Autodesk Inventor part; units mm, degrees
ref_plane "YZ Plane" through (0, 0, 0) normal (1, 0, 0) x (0, 1, 0)
ref_plane "XZ Plane" through (0, 0, 0) normal (0, 1, 0) x (-1, 0, 0)
ref_plane "XY Plane" through (0, 0, 0) normal (0, 0, 1) x (1, 0, 0)
sketch "Sketch3" plane through (0, 0, 0) normal (0, 1, 0) x (-1, 0, 0)
  circle A0 centre (0, 0) radius 13.5
  line L0 (-6.7499, 8.6501) -> (-1.7499, 8.6501)
  line L1 (-1.7499, 8.6501) -> (-1.7499, 7.1501)
  line L2 (-1.7499, 7.1501) -> (-6.7499, 7.1501)
  line L3 (-6.7499, 7.1501) -> (-6.7499, 8.6501)
  line L4 (-6.75, 5.45) -> (-1.7499, 5.45)
  line L5 (-1.7499, 5.45) -> (-1.7499, 3.95)
  line L6 (-1.7499, 3.95) -> (-6.75, 3.95)
  line L7 (-6.75, 3.95) -> (-6.75, 5.45)
  line L8 (-6.75, 2.0498) -> (-1.75, 2.0498)
  line L9 (-1.75, 2.0498) -> (-1.75, 0.5498)
  line L10 (-1.75, 0.5498) -> (-6.75, 0.5498)
  line L11 (-6.75, 0.5498) -> (-6.75, 2.0498)
  line L12 (-6.75, -1.2) -> (-1.75, -1.2)
  line L13 (-1.75, -1.2) -> (-1.75, -2.7)
  line L14 (-1.75, -2.7) -> (-6.75, -2.7)
  line L15 (-6.75, -2.7) -> (-6.75, -1.2)
  line L16 (-6.75, -4.4501) -> (-1.75, -4.4501)
  line L17 (-1.75, -4.4501) -> (-1.75, -5.9501)
  line L18 (-1.75, -5.9501) -> (-6.75, -5.9501)
  line L19 (-6.75, -5.9501) -> (-6.75, -4.4501)
  line L20 (1.9499, 7.1) -> (6.9499, 7.1)
  line L21 (6.9499, 7.1) -> (6.9499, 5.6)
  line L22 (6.9499, 5.6) -> (1.9499, 5.6)
  line L23 (1.9499, 5.6) -> (1.9499, 7.1)
  line L24 (1.9499, 3.95) -> (6.9499, 3.95)
  line L25 (6.9499, 3.95) -> (6.9499, 2.45)
  line L26 (6.9499, 2.45) -> (1.9499, 2.45)
  line L27 (1.9499, 2.45) -> (1.9499, 3.95)
  line L28 (1.9499, 0.5004) -> (6.9499, 0.5004)
  line L29 (6.9499, 0.5004) -> (6.9499, -0.9996)
  line L30 (6.9499, -0.9996) -> (1.9499, -0.9996)
  line L31 (1.9499, -0.9996) -> (1.9499, 0.5004)
  line L32 (1.9499, -2.7) -> (6.9499, -2.7)
  line L33 (6.9499, -2.7) -> (6.9499, -4.2)
  line L34 (6.9499, -4.2) -> (1.9499, -4.2)
  line L35 (1.9499, -4.2) -> (1.9499, -2.7)
  line L36 (1.9499, -6.1999) -> (6.9499, -6.1999)
  line L37 (6.9499, -6.1999) -> (6.9499, -7.6999)
  line L38 (6.9499, -7.6999) -> (1.9499, -7.6999)
  line L39 (1.9499, -7.6999) -> (1.9499, -6.1999)
  point P0 (-6.7499, 7.9001)
  point P1 (-6.75, 4.7)
  point P2 (-5.95, -5.2001)
  dimension "d3" = 27
  dimension "d4" = 5
  dimension "d5" = 1.5
  dimension "d6" = 1.5
  dimension "d7" = 5
  dimension "d8" = 1.5
  dimension "d9" = 5
  dimension "d10" = 1.5
  dimension "d11" = 5
  dimension "d12" = 1.5
  dimension "d13" = 0.8
  dimension "d14" = 5
  dimension "d15" = 1.5
  dimension "d16" = 5
  dimension "d17" = 1.5
  dimension "d18" = 5
  dimension "d19" = 1.5
  dimension "d20" = 5
  dimension "d21" = 1.5
  dimension "d22" = 1.5
extrude "Extrusion1" add sketch "Sketch3" along normal blind 5
sketch "Sketch4" plane through (0, 5, 0) normal (0, 1, 0) x (1, 0, 0)
  circle A0 centre (-10.8, -1.9) radius 0.75
  circle A1 centre (-10.8, 1.7) radius 0.75
  circle A2 centre (10.9, -1.85) radius 0.75
  circle A3 centre (10.9, 1.65) radius 0.75
  circle A4 centre (0.958, 9.985) radius 3
  point P0 (0, 0)
  dimension "d25" = 1.5
  dimension "d26" = 1.5
  dimension "d27" = 1.5
  dimension "d28" = 1.5
  dimension "d29" = 6
extrude "Extrusion2" cut sketch "Sketch4" against normal blind 5
sketch "Sketch5" plane through (0, 5, 0) normal (0, 1, 0) x (1, 0, 0)
  circle A0 centre (-10.8, -1.9) radius 0.75
  circle A1 centre (-10.8, -1.9) radius 1.25
  circle A2 centre (-10.8, 1.7) radius 0.75
  circle A3 centre (-10.8, 1.7) radius 1.25
  circle A4 centre (10.9, -1.85) radius 0.75
  circle A5 centre (10.9, -1.85) radius 1.25
  circle A6 centre (10.9, 1.65) radius 0.75
  circle A7 centre (10.9, 1.65) radius 1.25
  point P0 (0, 0)
  dimension "d33" = 2.5
  dimension "d34" = 2.5
  dimension "d35" = 2.5
  dimension "d36" = 2.5
extrude "Extrusion3" cut sketch "Sketch5" against normal blind 5 contours A0 | A1 | A2 | A3 | A4 | A5 | A6 | A7
properties part number "Seperator"
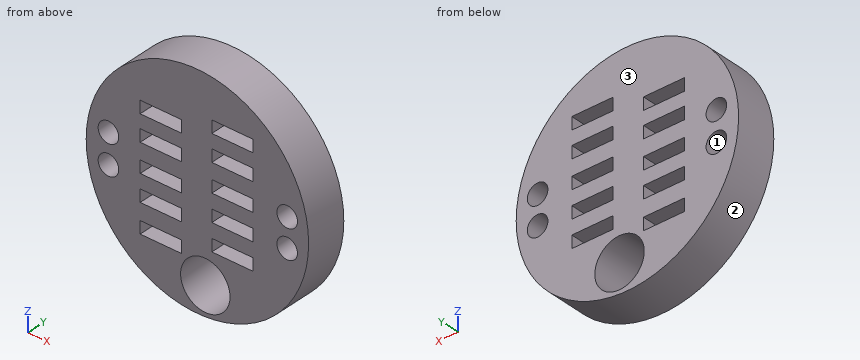
The model under review builds one solid part; all positions refer to its coordinate system, in mm. Face numbers are marked on the shaded views. Coordinates: 2 decimals unless noted, no trailing zeros. Write each loop counter-clockwise with the first axis right and the second up, starting at its lowest first coordinate (ties: lowest second). Pieces come first, ordered by that corner, then holes. Notation, with made-up numbers: (-29.5, -18.75) - (-2.5, -18.75) arc R14 ccw to (-2.5, -4.75) - close; hole circle Ø4 at (40.25, -26). An arc over 180 degrees is marked (long way). Answer as a JSON object with one key per item and string values. Group by question number.
1. To check wall thickness, follow probe 1 along Z at (x, y) = (-10.8, 3.6); probe 2 along Z at (x, y) = (10.9, 2.45); probe 3 along X at (y, z) = (2.9, 1.9). State the ranges of each line that lie inside material, in increasing order.
2. Mouldability with a two-part tool opening along X and no side actions: class the marked faces 1, 2 and 3 as pulls with the +X half, pulls with the -X half, needs draft (parallel to the pull), parting line crosses it, or undercut.
3. Add section A-A (x = -10.8). Give the boundary of the cut face in (y, z), plus the area to 3 significant figures.
4. Add section C-C (x = -0.25). Give the boundary of the cut face in (y, z), plus the area to 3 significant figures.
5. Add section D-D (y = 2). Give the number of separate pieces and of enclosed holes in the cut face, plus the area to 3 significant figures.
6. Clearance check with flat-ended pins moving along their axes: pin 1 Ø2 at (x, y) = (5, 4.5) entering from +Z; pin 2 Ø1.2 at (y, z) = (2.5, -7) entering from +X; pin 3 Ø0.8 at (y, z) = (3.5, 6.5) entering from +X; pin 4 Ø2 at (x, z) = (10.9, -1.65) entering from -Y. State where each tip first meets the part, or that it passes through.
7. Add section B-B (z = 3.5). Give the boundary of the cut face in (x, y).
Findings:
{
 "1": {"probe 1": "-8.1 to -2.95, -0.45 to 0.65, 3.15 to 8.1", "probe 2": "-7.96 to -2.9, -0.4 to 0.6, 3.1 to 7.96", "probe 3": "-13.37 to -12.05, -9.55 to 1.75, 6.75 to 9.65, 12.15 to 13.37"},
 "2": {"face 1": "undercut", "face 2": "parting line crosses it", "face 3": "needs draft"},
 "3": {"outline": "(0, -8.1) - (5, -8.1) - (5, -2.95) - (0, -2.95) - close; (0, -0.45) - (5, -0.45) - (5, 0.65) - (0, 0.65) - close; (0, 3.15) - (5, 3.15) - (5, 8.1) - (0, 8.1) - close", "area": "56.0 mm²"},
 "4": {"outline": "(0, -13.5) - (5, -13.5) - (5, -12.73) - (0, -12.73) - close; (0, -7.24) - (5, -7.24) - (5, 13.5) - (0, 13.5) - close", "area": "108 mm²"},
 "5": {"separate pieces": "1", "enclosed holes": "15", "area": "450 mm²"},
 "6": {"pin 1": "z = 12.89", "pin 2": "x = 11.89", "pin 3": "x = 12.04", "pin 4": "through"},
 "7": {"outline": "(-13.04, 0) - (-6.95, 0) - (-6.95, 5) - (-13.04, 5) - close; (-1.95, 0) - (13.04, 0) - (13.04, 5) - (-1.95, 5) - close"}
}
